For this review, use the dimensioned drawing (mm, ordinates from the lowest corner) and the shaded views. A direction names the side the tool comes from. Round coordinates to 2 decimals unless told otherwise and drop trailing zeros. Loops run counter-clockwise (first coordinate to the right, second up) from the corner with the lowest first, then second, coordinate; pieces in that order, holes last. Notation, with made-up numbers: (4.25, 56) - (48.25, 56) arc R26 ccw to (48.25, 87) - close; hole circle Ø5 at (9, 74.25). An arc over 180 degrees is marked (long way). Answer as CSV lines item,"result". Start each with the question number.
(1) Wall thickness on L1, parallel to Y at x = 40, z = 24; L2, parallel to Z at x = 41.5, y = 36; L3, parallel to Y at x = 185, z = 70: over which ranges is each line inside the solid? List them lowest first.
(2) Consider section C-C (z = 30.5). Give the boundary of the cut face in (x, y).
(3) Consider section B-B (x = 40). Give the boundary of the cut face in (y, z), and give its area (3 significant figures).
(4) Consider section D-D (y = 95). Give the boundary of the cut face in (x, z), and give its area (3 significant figures).
(5) Consider section A-A (y = 80). Give the boundary of the cut face in (x, z), and give its area (3 significant figures).
(6) For the marked faces 4 and 5, list the 3-axis set-ups (+Z, -Z, +X, -X, +Y, -Y) from which the entire face can be reached by the end or side of a thin tool; tool diameter is ignored.
(7) Mouldability with a two-part tool opening along Y and no side actions: class the marked faces 1, 2 and 3 as released by +Y, released by -Y, zero draft, split by the parting line, or undercut.
(8) For P1, Ø8, axis at y = 104.5, z = 55, coming from the -X side; P2, Ø3, axis at x = 61, y = 77.5, coming from the +Z side; P3, Ø1, axis at y = 101, z = 20, coming from the +X side, all flat-tipped, find the tip position at first contact; note any pin that passes through.
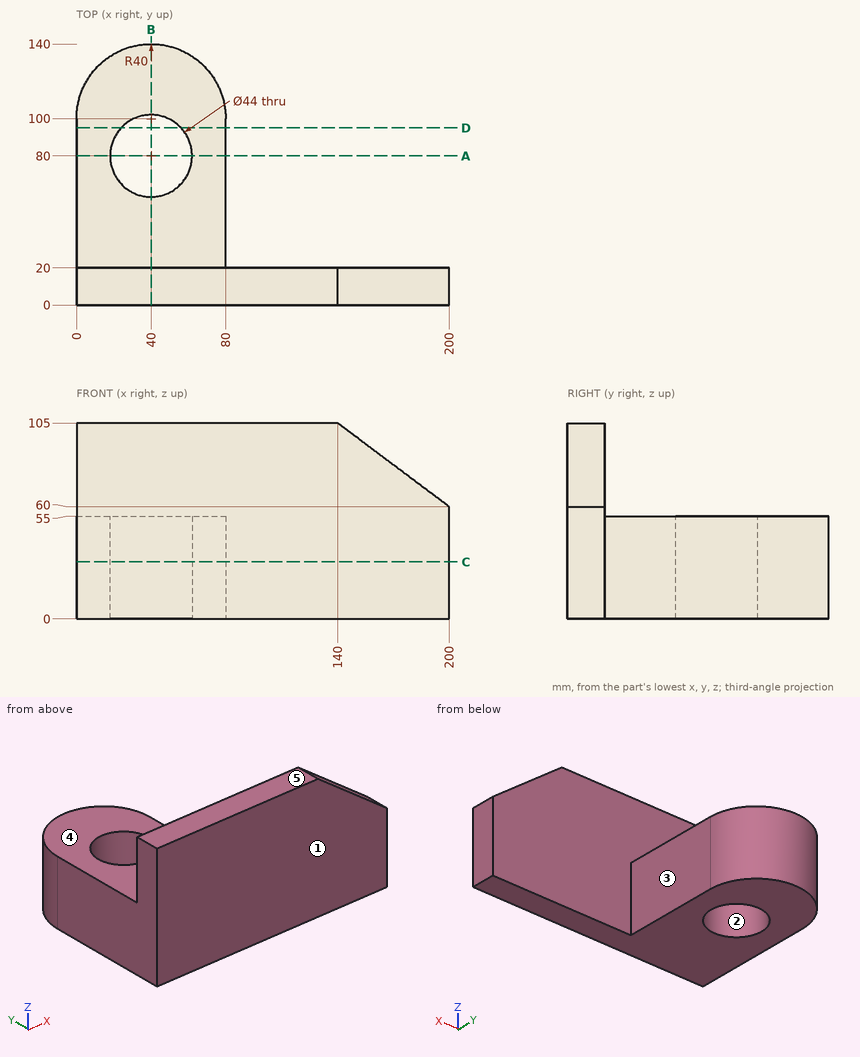
Determined:
1,L1,"y = 0 to 58, 102 to 140"
1,L2,"z = 0 to 55"
1,L3,"y = 0 to 20"
2,outline,"(0, 0) - (200, 0) - (200, 20) - (80, 20) - (80, 100) arc R40 ccw to (0, 100) - close; hole circle Ø44 at (40, 80)"
3,outline,"(0, 0) - (58, 0) - (58, 55) - (20, 55) - (20, 105) - (0, 105) - close; (102, 0) - (140, 0) - (140, 55) - (102, 55) - close"
3,area,"6,280 mm^2"
4,outline,"(0, 0) - (23.91, 0) - (23.91, 55) - (0, 55) - close; (56.09, 0) - (80, 0) - (80, 55) - (56.09, 55) - close"
4,area,"2,630 mm^2"
5,outline,"(0, 0) - (18, 0) - (18, 55) - (0, 55) - close; (62, 0) - (80, 0) - (80, 55) - (62, 55) - close"
5,area,"1,980 mm^2"
6,face 4,"+Z, +X, -X, +Y"
6,face 5,"+Z, +X, -X, +Y, -Y"
7,face 1,"released by -Y"
7,face 2,"undercut"
7,face 3,"zero draft"
8,P1,"stops at x = 0"
8,P2,"stops at z = 55"
8,P3,"stops at x = 80"
